Could you check a few things on this model? Use its own coordinates, in mm. A direction names the side the tool comes from. Give positions to 0.01 mm unless a question says otherwise; leave off trailing zeros. Write each loop counter-clockwise with the first axis right and the second up, starting at its lowest first coordinate (ties: lowest second). Pieces come first, ordered by that corner, then holes. Notation, with made-up numbers: M 9.5,-36.5 L 34.5,-36.5 A26 ccw 34.5,-4.5 Z; hole C -22.75,46 d1. An arc over 180 degrees is marked long. Answer as a JSON object with one key per item and string values. Group by question number.
```python
from build123d import *

# Parameters (mm, degrees)
F0_R       = 1.5
F0_R_2     = 2
F1_DEPTH   = 15
F2_W       = 5
F2_H       = 2.5
F3_DEPTH   = 30.001
F5_SIZE2   = 10
F5_SIZE    = 3
F5_2_SIZE2 = 10
F5_2_SIZE  = 3
F6_SIZE    = 0.49999
F4_R       = 3
F7_DEPTH   = 19.5
F8_SIZE    = 3
F9_W       = 15.6673565507
F9_H       = 12.20472157
F10_DEPTH  = 20


# Not quite as in the source:
# - a fillet or chamfer is up to 0.001 mm smaller than in the source, because OpenCascade refuses the exact size


with BuildPart() as f1:
    # F0 (on Front) → F1 (new body)
    with BuildSketch(Plane.XZ):
        Polygon((15, 0), (0, 0), (-15, 0), (-15, -50), (0, -50), (15, -50), align=None)
        with Locations((-12, -47)):
            Circle(F0_R, mode=Mode.SUBTRACT)
        with Locations((12, -47)):
            Circle(F0_R, mode=Mode.SUBTRACT)
        with Locations((-12, -23)):
            Circle(F0_R, mode=Mode.SUBTRACT)
        with Locations((-12, -9)):
            Circle(F0_R_2, mode=Mode.SUBTRACT)
        with Locations((12, -23)):
            Circle(F0_R, mode=Mode.SUBTRACT)
        with Locations((12, -9)):
            Circle(F0_R_2, mode=Mode.SUBTRACT)
    extrude(amount=F1_DEPTH)

    # F2 (on face) → F3 (cut, through all)
    with BuildSketch(Plane(origin=(-15, 0, 0), x_dir=(0, -1, 0), z_dir=(-1, 0, 0))):
        with Locations((12.5, -47.25)):
            Rectangle(F2_W, F2_H)
        with Locations((12.5, -43.25)):
            Rectangle(F2_W, F2_H)
        with Locations((12.5, -39.25)):
            Rectangle(F2_W, F2_H)
        with Locations((12.5, -35.25)):
            Rectangle(F2_W, F2_H)
        with Locations((12.5, -31.25)):
            Rectangle(F2_W, F2_H)
        with Locations((12.5, -27.25)):
            Rectangle(F2_W, F2_H)
        with Locations((12.5, -23.25)):
            Rectangle(F2_W, F2_H)
    extrude(amount=-F3_DEPTH, mode=Mode.SUBTRACT)

    # F5
    f5_edges = [f1.edges().sort_by_distance(p)[0] for p in [
        (-15, -7.5, 0),
    ]]
    f5_side = f1.faces().sort_by_distance((-15, -6.839623, -23.646226))[0]
    chamfer(f5_edges, length=F5_SIZE, length2=F5_SIZE2, reference=f5_side)

    # F5#2
    f5_2_edges = [f1.edges().sort_by_distance(p)[0] for p in [
        (15, -7.5, 0),
    ]]
    f5_2_side = f1.faces().sort_by_distance((15, -6.839623, -23.646226))[0]
    chamfer(f5_2_edges, length=F5_2_SIZE, length2=F5_2_SIZE2, reference=f5_2_side)

    # F6 (size 0.5 in the source; OpenCascade refuses exactly that, so slightly less here)
    f6_edges = [f1.edges().sort_by_distance(p)[0] for p in [
        (0, -15, 0),
        (10, -15, -1.5),
        (-10, -15, -1.5),
        (15, -15, -12.5),
        (-15, -15, -12.5),
        (14.059017, -15, -22),
        (-14.059017, -15, -22),
        (12, -15, -21.5),
        (-12, -15, -21.5),
        (0, -15, -22),
        (-14, -15, -9),
        (10, -15, -9),
    ]]
    chamfer(f6_edges, length=F6_SIZE)

    # F4 (on face) → F7 (join)
    with BuildSketch(Plane(origin=(0, 0, -50), x_dir=(1, 0, 0), z_dir=(0, 0, -1))):
        with Locations((0, 5)):
            Circle(F4_R)
    extrude(amount=F7_DEPTH)

    # F8
    f8_edges = [f1.edges().sort_by_distance(p)[0] for p in [
        (-3, -5, -69.5),
    ]]
    chamfer(f8_edges, length=F8_SIZE)

    # F9 (on Front) → F10 (join)
    with BuildSketch(Plane.XZ):
        with Locations((0, -58.2721680403)):
            Rectangle(F9_W, F9_H)
    extrude(amount=F10_DEPTH)


solid = f1.part
```
1) Please list where these lines run through material, in increasing order: line 1 along X through (y, z) = (-7.25, -23); line 2 along Z through (x, y) = (12.5, -5.25); line 3 along Z through (x, y) = (12, -6.25). Write a range as from..to.
2) We'd pull the mould along Z, two halves only. Please class faces 4 (the flat face through (0, -10, -64.375)), 5 (the flat face through (0, -10, -27)), 6 (the flat face through (-9.93, -7.15, -1.48)): released by +Z, released by -Z, zero draft, split by the parting line, or undercut.
3) If we section it at C-C, the plane z = -23: List the corners of the cut face in (x, y) for me, plus the area to 3 significant figures.
4) I'm going to push flat-ended pins straight in: pin 1 (3 mm diameter, centred on x = 13.5, z = -46.5, fed in from -Y); pin 2 (4 mm diameter, centred on x = -4, y = -13, fed in from -Z); pin 3 (1.5 mm diameter, centred on x = 14, y = -11.5, fed in from -Z). Where does each tip first touch, or does it pass through?
5) If we section it at A-A, the plane y = -8.75: List the corners of the cut face in (x, z) for me, plus the area to 3 significant figures.
6) If we section it at B-B, the plane z = -9: Give the number of separate pieces and of enclosed holes in the cut face, plus the area to 3 significant figures.
7) For faces 1 (the flat face through (0, -15, -37)), 2 (the cylindrical face through (-12.195, -5.537, -21.513)), 3 (the flat face through (-14, -12, -46)), which set-ups out of +Z, -Z, +X, -X, +Y, -Y let a thin tool reach every point of the face, with its end or its side?
Taken from the geometry:
{
 "1": {"line 1": "-15..-13.5, -10.5..10.5, 13.5..15", "line 2": "-50..-48.41, -45.59..-24.41, -21.59..-10.94, -7.06..-2.25", "line 3": "-50..-48.5, -45.5..-24.5, -21.5..-11, -7..-2.1"},
 "2": {"face 4": "released by -Z", "face 5": "undercut", "face 6": "released by +Z"},
 "3": {"outline": "M -15,-10 L -13.5,-10 L -13.5,0 L -15,0 Z; M -10.5,-10 L 10.5,-10 L 10.5,0 L -10.5,0 Z; M 13.5,-10 L 15,-10 L 15,0 L 13.5,0 Z", "area": "240 mm²"},
 "4": {"pin 1": "y = -15", "pin 2": "z = -64.37", "pin 3": "z = -50"},
 "5": {"outline": "M -15,-50 L 15,-50 L 15,-3 L 5,0 L -5,0 L -15,-3 Z; M -7.83,-64.37 L 7.83,-64.37 L 7.83,-52.17 L -7.83,-52.17 Z; hole C -12,-9 d4; hole C -12,-47 d3; hole C -12,-23 d3; hole C 12,-9 d4; hole C 12,-47 d3; hole C 12,-23 d3", "area": "1,610 mm²"},
 "6": {"separate pieces": "3", "enclosed holes": "0", "area": "329 mm²"},
 "7": {"face 1": "+Z, +X, -X, -Y", "face 2": "+Y, -Y", "face 3": "+X, -X, -Y"}
}
